Check sheet for the drawn part. Datum: minimum x, y, z corner. Units: mm. A direction names the side the tool comes from. Give positions to 0.01 mm unless a question says otherwise; leave off trailing zeros. Write each loop counter-clockwise with the first axis right and the second up, starting at its lowest first coordinate (ties: lowest second). Pieces come first, ordered by that corner, then holes.
(1) Cross-section at B-B (y = 9.75). Record the boundary of the cut face in (x, z).
(2) Cross-section at A-A (z = 9.25). Record the boundary of the cut face in (x, y).
(3) Tool access check on the marked faces 1, 2 and 3. Record the directions out of +Z, -Z, +X, -X, +Y, -Y that give a thin tool (end or side, any length) a straight path to the whole face; none if there is none.
(4) Mould release check, pull along Y, two halves, no side actions. Record for the marked faces 4, 5, 6 and 7: +Y half, -Y half, draft (parallel to the pull), parting line (faces both ways), or undercut.
(5) Cross-section at C-C (x = 11.25). Record the boundary of the cut face in (y, z).
(6) Thickness scan on line 1 along Y through (x, z) = (17.75, 3); line 2 along Y through (x, z) = (10, 6.75); line 3 along X through (y, z) = (14, 2). Record the ranges inside material, lowest first.
(7) Depth check by flat-ended pin: P1, Ø3, axis at x = 8.5, z = 3, coming from the -Y side. Enter the tip coordinate at first touch or a pass-through.
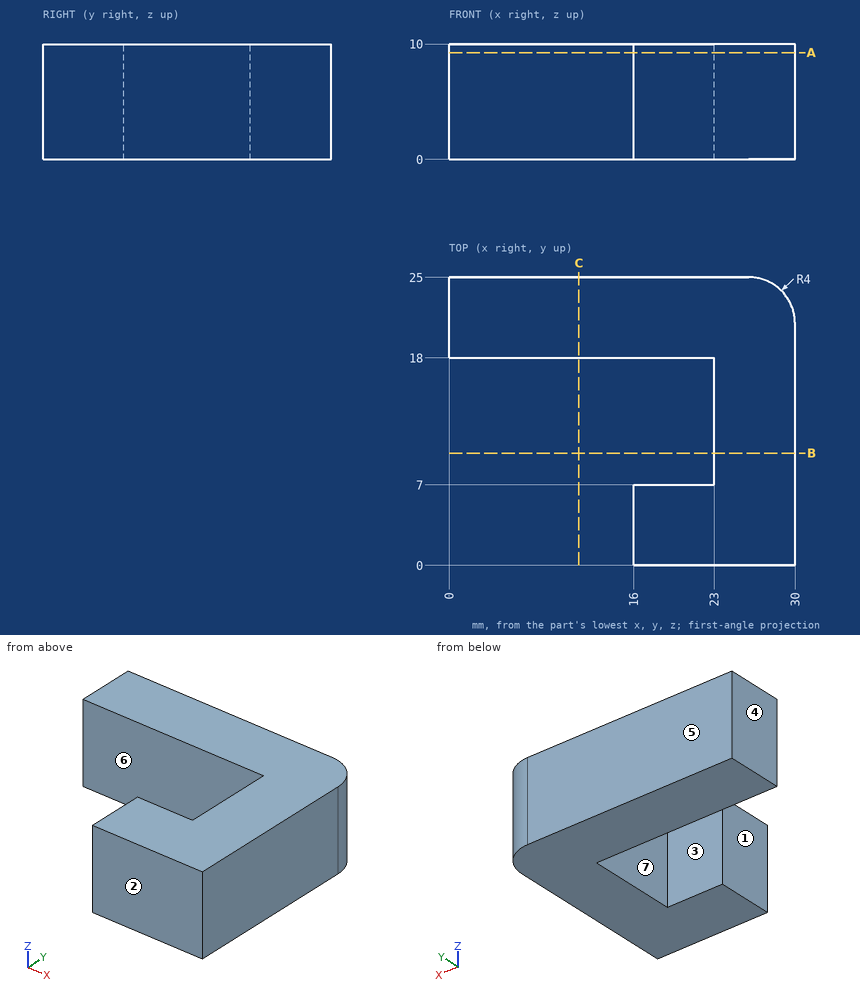
Reply:
1. outline: (23, 0) - (30, 0) - (30, 10) - (23, 10) - close
2. outline: (0, 18) - (23, 18) - (23, 7) - (16, 7) - (16, 0) - (30, 0) - (30, 21) arc R4 ccw to (26, 25) - (0, 25) - close
3. face 1: +Z, -Z, -X, -Y
3. face 2: +Z, -Z, +X, -X, -Y
3. face 3: +Z, -Z, -X
4. face 4: draft
4. face 5: +Y half
4. face 6: undercut
4. face 7: undercut
5. outline: (18, 0) - (25, 0) - (25, 10) - (18, 10) - close
6. line 1: y = 0 to 7, 18 to 25
6. line 2: y = 18 to 25
6. line 3: x = 23 to 30
7. P1: stops at y = 18
